Read the model definition and answer for the solid it produces. Units are mm, in the model's axes. A direction names the side the tool comes from. Round coordinates to 2 decimals unless told otherwise and drop trailing zeros. Order: outer loops, then holes, each group sorted by start corner. A loop starts at its lowest first (then second) coordinate and runs counter-clockwise, first axis right, second up.
from build123d import *

# Parameters (mm, degrees)
SKETCH_1_W          = 8
SKETCH_1_H          = 2.9
EXTRUDE_1_DEPTH     = 5.61
SKETCH_2_W          = 0.25
SKETCH_2_H          = 0.25
EXTRUDE_2_DEPTH     = 2.29
FILLET_2_R          = 0.5
CUT_EXTRUDE_1_DEPTH = 2
EXTRUDE_3_DEPTH     = 1


with BuildPart() as part:
    # 草图1 → 凸台-拉伸1 (new body)
    with BuildSketch(Plane(origin=(0, 0, 0), x_dir=(1, 0, 0), z_dir=(0, 1, 0))):
        Rectangle(SKETCH_1_W, SKETCH_1_H)
    extrude(amount=EXTRUDE_1_DEPTH)

    # 草图2 → 凸台-拉伸2 (add)
    with BuildSketch(Plane.XZ):
        with Locations((-1.3, 0.5)):
            Rectangle(SKETCH_2_W, SKETCH_2_H)
        with Locations((1.3, 0.5)):
            Rectangle(SKETCH_2_W, SKETCH_2_H)
        with Locations((0, 0.5)):
            Rectangle(SKETCH_2_W, SKETCH_2_H)
        with Locations((-0.65, -0.5)):
            Rectangle(SKETCH_2_W, SKETCH_2_H)
        with Locations((0.65, -0.5)):
            Rectangle(SKETCH_2_W, SKETCH_2_H)
    extrude(amount=EXTRUDE_2_DEPTH)

    # 圆角2
    fillet_2_edges = [part.edges().sort_by_distance(p)[0] for p in [
        (-4, 2.805, -1.45),
        (4, 2.805, -1.45),
        (4, 2.805, 1.45),
        (-4, 2.805, 1.45),
    ]]
    fillet(fillet_2_edges, radius=FILLET_2_R)

    # 草图3 → 切除-拉伸1 (cut)
    with BuildSketch(Plane(origin=(0, 5.61, 0), x_dir=(1, 0, 0), z_dir=(0, 1, 0))):
        with BuildLine():
            Line((3.75, -0.95), (3.75, 0.95))
            ThreePointArc((3.75, 0.95), (3.676776695, 1.126776695), (3.5, 1.2))
            Line((3.5, 1.2), (-3.5, 1.2))
            ThreePointArc((-3.5, 1.2), (-3.676776695, 1.126776695), (-3.75, 0.95))
            Line((-3.75, 0.95), (-3.75, -0.95))
            ThreePointArc((-3.75, -0.95), (-3.676776695, -1.126776695), (-3.5, -1.2))
            Line((-3.5, -1.2), (3.5, -1.2))
            ThreePointArc((3.5, -1.2), (3.676776695, -1.126776695), (3.75, -0.95))
        make_face()
    extrude(amount=-CUT_EXTRUDE_1_DEPTH, mode=Mode.SUBTRACT)

    # 草图4 → 凸台-拉伸3 (add)
    with BuildSketch(Plane(origin=(0, 3.61, 0), x_dir=(1, 0, 0), z_dir=(0, 1, 0))):
        with BuildLine():
            Line((-1.75, 0.55), (1.75, 0.55))
            ThreePointArc((1.75, 0.55), (2.125, 0.175), (1.75, -0.2))
            Line((1.75, -0.2), (-1.75, -0.2))
            ThreePointArc((-1.75, -0.2), (-2.125, 0.175), (-1.75, 0.55))
        make_face()
    extrude(amount=EXTRUDE_3_DEPTH)


solid = part.part
Q1. For faces 4 (the face through (-4, 3, 0)), 5 (the face through (3.75, 5, 0)), determine the directions among +Z, -Z, +X, -X, +Y, -Y from which every point of the face is accessible in a straight line to the end or side of a thin tool.
Outcome:
face 4: +Z, -Z, -X, +Y, -Y
face 5: +Y
Q2. A cutting plane is placed at A-A, the plane y = 4.5. Give the vertices of the cut face in (x, z) (3 decimals), plus the area to 3 significant figures.
Outcome:
outline: (-4, -0.95) arc R0.5 ccw to (-3.5, -1.45) - (3.5, -1.45) arc R0.5 ccw to (4, -0.95) - (4, 0.95) arc R0.5 ccw to (3.5, 1.45) - (-3.5, 1.45) arc R0.5 ccw to (-4, 0.95) - close; (-1.75, -0.55) - (1.75, -0.55) arc R0.375 ccw to (1.75, 0.2) - (-1.75, 0.2) arc R0.375 ccw to start; hole (-3.75, -0.95) arc R0.25 ccw to (-3.5, -1.2) - (3.5, -1.2) arc R0.25 ccw to (3.75, -0.95) - (3.75, 0.95) arc R0.25 ccw to (3.5, 1.2) - (-3.5, 1.2) arc R0.25 ccw to (-3.75, 0.95) - close
area: 8.11 mm2
Q3. For a pull along X with two mould halves and no side action, classify faces 1 (the face through (0, 5, -1.2)), 2 (the face through (4, 3, 0)), 3 (the face through (0, 3, 1.45)) as released by +X, released by -X, zero draft, split by the parting line, or undercut.
Outcome:
face 1: undercut
face 2: released by +X
face 3: zero draft
Q4. Straight lines are drawn through the part: probe 1 along X at (y, z) = (4.5, 0.65); probe 2 along Y at (x, z) = (1, 0.65); probe 3 along Y at (x, z) = (0.5, -1.3). For each, find the intervals that lie inside material, in ascending order.
Outcome:
probe 1: x = -4 to -3.75, 3.75 to 4
probe 2: y = 0 to 3.61
probe 3: y = 0 to 5.61
Q5. A cutting plane is placed at D-D, the plane y = -1. Give the vertices of the cut face in (x, z) (3 decimals).
Outcome:
outline: (-1.425, 0.375) - (-1.175, 0.375) - (-1.175, 0.625) - (-1.425, 0.625) - close; (-0.775, -0.625) - (-0.525, -0.625) - (-0.525, -0.375) - (-0.775, -0.375) - close; (-0.125, 0.375) - (0.125, 0.375) - (0.125, 0.625) - (-0.125, 0.625) - close; (0.525, -0.625) - (0.775, -0.625) - (0.775, -0.375) - (0.525, -0.375) - close; (1.175, 0.375) - (1.425, 0.375) - (1.425, 0.625) - (1.175, 0.625) - close
Q6. A cutting plane is placed at B-B, the plane z = -0.8. Give the vertices of the cut face in (x, y), plus the area to 3 significant figures.
Outcome:
outline: (-4, 0) - (4, 0) - (4, 5.61) - (3.75, 5.61) - (3.75, 3.61) - (-3.75, 3.61) - (-3.75, 5.61) - (-4, 5.61) - close
area: 29.9 mm2
Q7. A cutting plane is placed at C-C, the plane x = -3. Give the vertices of the cut face in (y, z), plus the area to 3 significant figures.
Outcome:
outline: (0, -1.45) - (5.61, -1.45) - (5.61, -1.2) - (3.61, -1.2) - (3.61, 1.2) - (5.61, 1.2) - (5.61, 1.45) - (0, 1.45) - close
area: 11.5 mm2
